Work out the finished part from the listing and answer in its coordinate system (mm). Face numbers are marked on the shaded views. Round coordinates to 2 decimals unless told otherwise and drop trailing zeros. Order: outer loops, then holes, each group sorted by start corner. A loop starts at its lowest first (then second) coordinate and runs counter-clockwise, first axis right, second up. Notation, with made-up numbers: (36.5, 25) - (69.5, 25) arc R33 ccw to (69.5, 62) - close; hole circle Ø11 at (87.5, 71.5). An arc over 180 degrees is marked (long way). Put each result on its own line as item: value.
```python
from build123d import *

# Parameters (mm, degrees)
F1_DEPTH = 12.7
F3_DEPTH = 25.4
F4_R     = 0.508


with BuildPart() as f1:
    # F0 (on Front) → F1 (new body)
    with BuildSketch(Plane.XZ):
        with BuildLine():
            ThreePointArc((-3.672035, -1.016), (-3.81, 0), (-3.672035, 1.016))
            Line((-3.672035, 1.016), (-4.717841, 1.016))
            ThreePointArc((-4.717841, 1.016), (-4.826, 0), (-4.717841, -1.016))
            Line((-4.717841, -1.016), (-3.672035, -1.016))
        make_face()
    extrude(amount=F1_DEPTH)

    # F2 (on Right) → F3 (cut)
    with BuildSketch(Plane.YZ):
        with BuildLine():
            Line((-12.7, 1.016), (-12.7, 0))
            Line((-12.7, 0), (-12.7, -1.016))
            Line((-12.7, -1.016), (-9.525, -1.016))
            ThreePointArc((-9.525, -1.016), (-10.541, 0), (-9.525, 1.016))
            Line((-9.525, 1.016), (-12.7, 1.016))
        make_face()
        with BuildLine():
            ThreePointArc((-3.175, 1.016), (-2.159, 0), (-3.175, -1.016))
            Line((-3.175, -1.016), (0, -1.016))
            Line((0, -1.016), (0, 1.016))
            Line((0, 1.016), (-3.175, 1.016))
        make_face()
    extrude(amount=-F3_DEPTH, mode=Mode.SUBTRACT)

    # F4
    f4_edges = [f1.edges().sort_by_distance(p)[0] for p in [
        (-4.717841, -6.35, 1.016),
    ]]
    fillet(f4_edges, radius=F4_R)


solid = f1.part
```
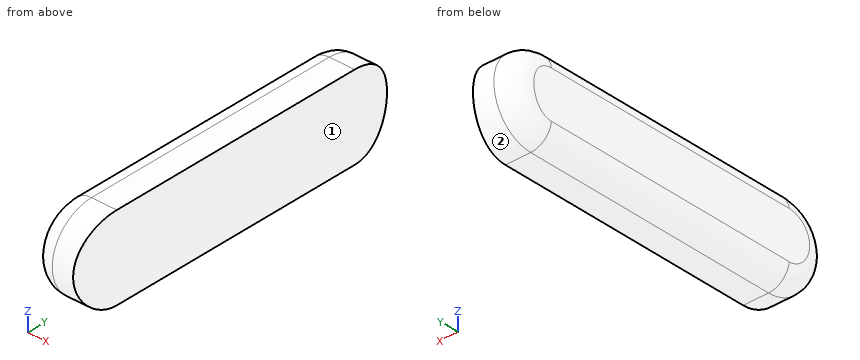
1) Straight lines are drawn through the part: L1, parallel to X at y = -8, z = -0.05; L2, parallel to Z at x = -3.9, y = -3; L3, parallel to Y at x = -4.15, z = 0.35. For each, find the intervals that lie inside material, in ascending order. Write a range as from..to.
Findings below:
L1: x = -4.83..-3.81
L2: z = -1..1
L3: y = -10.48..-2.22
2) For a pull along Z with two mould halves and no side action, classify the marked faces 1 and 2 as pulls with the +Z half, pulls with the -Z half, needs draft (parallel to the pull), parting line crosses it, or undercut.
Findings below:
face 1: undercut
face 2: parting line crosses it
3) A cutting plane is placed at A-A on y = -5. Write down the section's boundary in (x, z).
Findings below:
outline: (-4.79, -0.57) arc R0.51 ccw to (-4.29, -1.02) - (-3.67, -1.02) arc R3.81 cw to (-3.67, 1.02) - (-4.29, 1.02) arc R0.51 ccw to (-4.79, 0.57) arc R4.83 ccw to start
